Check sheet for the modelled part. Datum: model origin and axes. Units: mm. Round coordinates to 2 decimals unless told otherwise and drop trailing zeros. Order: outer loops, then holes, each group sorted by start corner. A loop starts at its lowest first (then second) coordinate and runs counter-clockwise, first axis right, second up. Notation, with made-up numbers: (60.25, 68) -> (105.25, 68) arc R23 ccw to (105.25, 80) -> close; hole circle Ø4 at (-33, -25). An arc over 180 degrees is marked (long way). Use CSV: the item, a comma, the result in double quotes.
```python
from build123d import *

# Parameters (mm, degrees)
BOSS_EXTRUDE1_DEPTH  = 3.175
SKETCH3_W            = 107.95
SKETCH3_H            = 3.175
CUT_EXTRUDE2_DEPTH   = 549.843544419
FILLET1_R            = 1.5875
CUT_EXTRUDE1_DEPTH   = 549.843544419
LPATTERN1_COUNT      = 3
LPATTERN1_PITCH      = 101.6
MIRROR1_COPY_1_DEPTH = 549.843544419
MIRROR1_COPY_2_DEPTH = 549.843544419
SKETCH4_R            = 1.5875
SKETCH4_R_2          = 57.5
CUT_EXTRUDE3_DEPTH   = 549.843544419


with BuildPart() as part:
    # Sketch1 → Boss-Extrude1 (new body)
    with BuildSketch(Plane(origin=(0, 0, 0), x_dir=(1, 0, 0), z_dir=(0, 1, 0))):
        Polygon((401.6375, 0), (447.675, 0), (447.675, 317.5), (0, 317.5), (0, 0), (46.0375, 0), (46.0375, -3.175), (401.6375, -3.175), align=None)
    extrude(amount=BOSS_EXTRUDE1_DEPTH)

    # Sketch3 → Cut-Extrude2 (cut, through all)
    with BuildSketch(Plane(origin=(0, 3.175, 0), x_dir=(1, 0, 0), z_dir=(0, 1, 0))):
        with Locations((122.2375, 315.9125)):
            Rectangle(SKETCH3_W, SKETCH3_H)
        with Locations((325.4375, 315.9125)):
            Rectangle(SKETCH3_W, SKETCH3_H)
    extrude(amount=-CUT_EXTRUDE2_DEPTH, mode=Mode.SUBTRACT)

    # Fillet1
    fillet1_edges = [part.edges().sort_by_distance(p)[0] for p in [
        (379.4125, 1.5875, -317.5),
        (271.4625, 1.5875, -317.5),
        (176.2125, 1.5875, -317.5),
        (68.2625, 1.5875, -317.5),
        (379.4125, 1.5875, -314.325),
        (271.4625, 1.5875, -314.325),
        (176.2125, 1.5875, -314.325),
        (68.2625, 1.5875, -314.325),
        (447.675, 1.5875, -317.5),
        (447.675, 1.5875, 0),
        (0, 1.5875, 0),
        (0, 1.5875, -317.5),
        (401.6375, 1.5875, 3.175),
        (401.6375, 1.5875, 0),
        (46.0375, 1.5875, 3.175),
        (46.0375, 1.5875, 0),
    ]]
    fillet(fillet1_edges, radius=FILLET1_R - 0.0001)  # a hair under: the kernel refuses the full size

    # Sketch2 → Cut-Extrude1 (cut, through all)
    with BuildSketch(Plane(origin=(0, 3.175, 0), x_dir=(1, 0, 0), z_dir=(0, 1, 0))):
        with BuildLine():
            Line((10.795, 258.047403349), (10.795, 260.35))
            ThreePointArc((10.795, 260.35), (12.7, 262.255), (14.605, 260.35))
            Line((14.605, 260.35), (14.605, 258.047403349))
            ThreePointArc((14.605, 258.047403349), (12.7, 248.92), (10.795, 258.047403349))
        make_face()
    cut_extrude1 = extrude(amount=-CUT_EXTRUDE1_DEPTH, mode=Mode.SUBTRACT)

    # LPattern1: Cut-Extrude1 ×3
    with Locations(*[(0, 0, i * LPATTERN1_PITCH) for i in range(1, LPATTERN1_COUNT)]):
        add(cut_extrude1, mode=Mode.SUBTRACT)

    # Mirror1: Cut-Extrude1 across plane
    add(cut_extrude1.mirror(Plane.ZY.offset(-223.8375)), mode=Mode.SUBTRACT)

    # Mirror1 copy 1 sketch → Mirror1 copy 1 (cut, through all)
    with BuildSketch(Plane(origin=(447.675, 3.175, 101.6), x_dir=(-1, 0, 0), z_dir=(0, 1, 0))):
        with BuildLine():
            Line((10.795, -258.047403349), (10.795, -260.35))
            ThreePointArc((10.795, -260.35), (12.7, -262.255), (14.605, -260.35))
            Line((14.605, -260.35), (14.605, -258.047403349))
            ThreePointArc((14.605, -258.047403349), (12.7, -248.92), (10.795, -258.047403349))
        make_face()
    extrude(amount=-MIRROR1_COPY_1_DEPTH, mode=Mode.SUBTRACT)

    # Mirror1 copy 2 sketch → Mirror1 copy 2 (cut, through all)
    with BuildSketch(Plane(origin=(447.675, 3.175, 203.2), x_dir=(-1, 0, 0), z_dir=(0, 1, 0))):
        with BuildLine():
            Line((10.795, -258.047403349), (10.795, -260.35))
            ThreePointArc((10.795, -260.35), (12.7, -262.255), (14.605, -260.35))
            Line((14.605, -260.35), (14.605, -258.047403349))
            ThreePointArc((14.605, -258.047403349), (12.7, -248.92), (10.795, -258.047403349))
        make_face()
    extrude(amount=-MIRROR1_COPY_2_DEPTH, mode=Mode.SUBTRACT)

    # Sketch4 → Cut-Extrude3 (cut, through all)
    with BuildSketch(Plane(origin=(0, 3.175, 0), x_dir=(1, 0, 0), z_dir=(0, 1, 0))):
        with Locations(Location((62.70625, 276.225, 0), (0, 0, 270))):
            Circle(SKETCH4_R)
        with Locations(Location((169.06875, 276.225, 0), (0, 0, 270))):
            Circle(SKETCH4_R)
        with Locations(Location((169.06875, 169.8625, 0), (0, 0, 270))):
            Circle(SKETCH4_R)
        with Locations(Location((62.70625, 169.8625, 0), (0, 0, 270))):
            Circle(SKETCH4_R)
        with Locations(Location((115.8875, 223.04375, 0), (0, 0, 270))):
            Circle(SKETCH4_R_2)
    extrude(amount=-CUT_EXTRUDE3_DEPTH, mode=Mode.SUBTRACT)


solid = part.part
```
Q1. Sectioned sample at B-B, the plane x = 126.5. Enter the section's corners in (y, z) (3 decimals), then the cut area to 3 significant figures.
Result sheet:
outline,"(0, -314.325) -> (3.175, -314.325) -> (3.175, -279.556) -> (0, -279.556) -> close; (0, -166.532) -> (3.175, -166.532) -> (3.175, 3.175) -> (0, 3.175) -> close"
area,"649 mm^2"
Q2. Sectioned sample at A-A, the plane z = -193.5. Enter the section's corners in (x, y) (3 decimals).
Result sheet:
outline,"(0, 0) -> (66.558, 0) -> (66.558, 3.175) -> (0, 3.175) -> close; (165.217, 0) -> (447.675, 0) -> (447.675, 3.175) -> (165.217, 3.175) -> close"
Q3. Sectioned sample at C-C, the plane y = 2.45. State how many separate pieces and enclosed holes the cut face has, then the cut area to 3 significant figures.
Result sheet:
separate pieces,"1"
enclosed holes,"11"
area,"132,000 mm^2"
Q4. Mould release check, pull along Z, two halves, no side actions. Record for faces 1 (the face through (221, 3.175, -159)), 2 (the face through (434.793, 1.61, -147.323)): pulls with the +Z half, pulls with the -Z half, needs draft (parallel to the pull), parting line crosses it, or undercut.
Result sheet:
face 1,"needs draft"
face 2,"undercut"
Q5. Scan lines: L1, parallel to Z at x = 12.7, y = 2.4 (3 decimals); L2, parallel to X at y = 1.8, z = -153 (3 decimals); L3, parallel to X at y = 1.4, z = -55 (3 decimals). Record each from-to range of solid material in increasing order.
Result sheet:
L1,"z = -317.5 to -262.255, -248.92 to -160.655, -147.32 to -59.055, -45.72 to 0"
L2,"x = 0 to 8.027, 17.373 to 430.302, 439.648 to 447.675"
L3,"x = 0 to 10.795, 14.605 to 433.07, 436.88 to 447.675"
